Can you work these out from the model? Positions are in its coordinate system, mm. Face numbers are marked on the shaded views. A direction names the side the tool comes from. Round coordinates to 2 decimals unless told otherwise and drop trailing zeros. Loops run counter-clockwise (first coordinate to the right, second up) from the corner with the lowest first, then second, coordinate; pieces in that order, holes last. Notation, with made-up numbers: (-33, 72.5) - (-5, 72.5) arc R12 cw to (-5, 79.5) - close; hole circle Ø5 at (89.5, 15.25). An arc over 180 degrees is marked (long way). Answer as CSV lines item,"result".
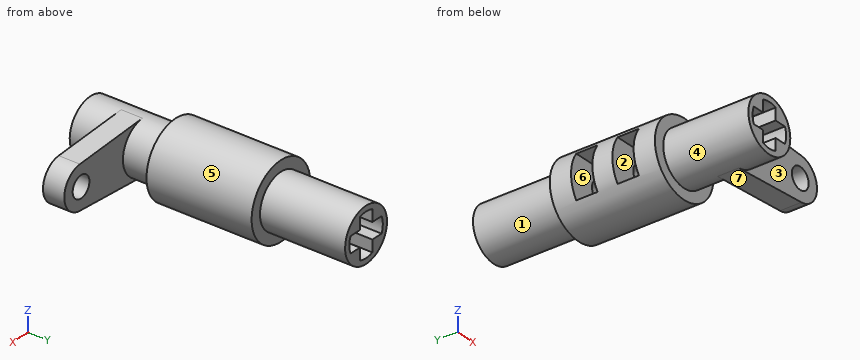
```python
from build123d import *

# Parameters (mm, degrees)
SKETCH_1_R           = 2.5
EXTRUDE_1_DEPTH      = 25.88
EXTRUDE_START        = 3
SKETCH_2_R           = 1
EXTRUDE_2_DEPTH      = 2
CUT_EXTRUDE_1_DEPTH  = 4
CUT_EXTRUDE_START    = 21.88
CUT_EXTRUDE_2_DEPTH  = 4
SKETCH_6_R           = 0.25
CUT_EXTRUDE_3_DEPTH  = 0.25
CUT_EXTRUDE_START_2  = 4.25
SKETCH_7_R           = 0.25
CUT_EXTRUDE_4_DEPTH  = 0.25
EXTRUDE_START_2      = 8
SKETCH_17_R          = 3.5
EXTRUDE_5_DEPTH      = 9.88
SKETCH_18_R          = 1
CUT_EXTRUDE_11_DEPTH = 10
CUT_EXTRUDE_START_3  = 15.88
SKETCH_19_R          = 1
CUT_EXTRUDE_12_DEPTH = 10
SKETCH_22_W          = 4
SKETCH_22_H          = 2
CUT_EXTRUDE_13_DEPTH = 10
CUT_EXTRUDE_14_DEPTH = 2
CUT_EXTRUDE_START_4  = 12
CUT_EXTRUDE_15_DEPTH = 2
SKETCH_25_R          = 1
CUT_EXTRUDE_16_DEPTH = 28.789825476


with BuildPart() as part:
    # 草图1 → 凸台-拉伸1 (new body)
    with BuildSketch(Plane(origin=(0, 0, 0), x_dir=(1, 0, 0), z_dir=(0, 1, 0))):
        with Locations(Location((0, 0, 0), (0, 0, 270))):
            Circle(SKETCH_1_R)
    extrude(amount=EXTRUDE_1_DEPTH)

    # 草图2 → 凸台-拉伸2 (add)
    with BuildSketch(Plane(origin=(0, 0, 0), x_dir=(1, 0, 0), z_dir=(0, 1, 0)).offset(EXTRUDE_START)):
        with BuildLine():
            Line((0.166666667, 2.494438258), (7.633333333, 1.995550606))
            ThreePointArc((7.633333333, 1.995550606), (9.5, 0), (7.633333333, -1.995550606))
            Line((7.633333333, -1.995550606), (0.166666667, -2.494438258))
            ThreePointArc((0.166666667, -2.494438258), (-2.5, 0), (0.166666667, 2.494438258))
        make_face()
        with Locations(Location((7.5, 0, 0), (0, 0, 270))):
            Circle(SKETCH_2_R, mode=Mode.SUBTRACT)
    extrude(amount=EXTRUDE_2_DEPTH)

    # 草图3 → 切除-拉伸1 (cut)
    with BuildSketch(Plane(origin=(0, 0, 0), x_dir=(1, 0, 0), z_dir=(0, 1, 0))):
        with BuildLine():
            Line((-1.854049622, -0.75), (-0.75, -0.75))
            Line((-0.75, -0.75), (-0.75, -1.854049622))
            ThreePointArc((-0.75, -1.854049622), (0, -2), (0.75, -1.854049622))
            Line((0.75, -1.854049622), (0.75, -0.75))
            Line((0.75, -0.75), (1.854049622, -0.75))
            ThreePointArc((1.854049622, -0.75), (2, 0), (1.854049622, 0.75))
            Line((1.854049622, 0.75), (0.75, 0.75))
            Line((0.75, 0.75), (0.75, 1.854049622))
            ThreePointArc((0.75, 1.854049622), (0, 2), (-0.75, 1.854049622))
            Line((-0.75, 1.854049622), (-0.75, 0.75))
            Line((-0.75, 0.75), (-1.854049622, 0.75))
            ThreePointArc((-1.854049622, 0.75), (-2, 0), (-1.854049622, -0.75))
        make_face()
    extrude(amount=CUT_EXTRUDE_1_DEPTH, mode=Mode.SUBTRACT)

    # 草图5 → 切除-拉伸2 (cut)
    with BuildSketch(Plane(origin=(0, 0, 0), x_dir=(1, 0, 0), z_dir=(0, 1, 0)).offset(CUT_EXTRUDE_START)):
        with BuildLine():
            Line((1.854049622, 0.75), (0.75, 0.75))
            Line((0.75, 0.75), (0.75, 1.854049622))
            ThreePointArc((0.75, 1.854049622), (0, 2), (-0.75, 1.854049622))
            Line((-0.75, 1.854049622), (-0.75, 0.75))
            Line((-0.75, 0.75), (-1.854049622, 0.75))
            ThreePointArc((-1.854049622, 0.75), (-2, 0), (-1.854049622, -0.75))
            Line((-1.854049622, -0.75), (-0.75, -0.75))
            Line((-0.75, -0.75), (-0.75, -1.854049622))
            ThreePointArc((-0.75, -1.854049622), (0, -2), (0.75, -1.854049622))
            Line((0.75, -1.854049622), (0.75, -0.75))
            Line((0.75, -0.75), (1.854049622, -0.75))
            ThreePointArc((1.854049622, -0.75), (2, 0), (1.854049622, 0.75))
        make_face()
    extrude(amount=CUT_EXTRUDE_2_DEPTH, mode=Mode.SUBTRACT)

    # 草图6 → 切除-拉伸3 (cut)
    with BuildSketch(Plane(origin=(0, 0, 0), x_dir=(1, 0, 0), z_dir=(0, 1, 0)).offset(CUT_EXTRUDE_START)):
        with Locations(Location((0.75, 0, 0), (0, 0, 270))):
            Circle(SKETCH_6_R)
    extrude(amount=-CUT_EXTRUDE_3_DEPTH, mode=Mode.SUBTRACT)

    # 草图7 → 切除-拉伸4 (cut)
    with BuildSketch(Plane(origin=(0, 0, 0), x_dir=(1, 0, 0), z_dir=(0, 1, 0)).offset(CUT_EXTRUDE_START_2)):
        with Locations(Location((0.75, 0, 0), (0, 0, 270))):
            Circle(SKETCH_7_R)
    extrude(amount=-CUT_EXTRUDE_4_DEPTH, mode=Mode.SUBTRACT)

    # 草图17 → 凸台-拉伸5 (add)
    with BuildSketch(Plane(origin=(0, 0, 0), x_dir=(1, 0, 0), z_dir=(0, 1, 0)).offset(EXTRUDE_START_2)):
        with Locations(Location((0, 0, 0), (0, 0, 270))):
            Circle(SKETCH_17_R)
    extrude(amount=EXTRUDE_5_DEPTH)

    # 草图18 → 切除-拉伸11 (cut)
    with BuildSketch(Plane(origin=(0, 0, 0), x_dir=(1, 0, 0), z_dir=(0, 1, 0))):
        with Locations(Location((0, 0, 0), (0, 0, 270))):
            Circle(SKETCH_18_R)
    extrude(amount=CUT_EXTRUDE_11_DEPTH, mode=Mode.SUBTRACT)

    # 草图19 → 切除-拉伸12 (cut)
    with BuildSketch(Plane(origin=(0, 0, 0), x_dir=(1, 0, 0), z_dir=(0, 1, 0)).offset(CUT_EXTRUDE_START_3)):
        with Locations(Location((0, 0, 0), (0, 0, 270))):
            Circle(SKETCH_19_R)
    extrude(amount=CUT_EXTRUDE_12_DEPTH, mode=Mode.SUBTRACT)

    # 草图22 → 切除-拉伸13 (cut)
    with BuildSketch(Plane(origin=(0, 0, 0), x_dir=(0, 0, -1), z_dir=(1, 0, 0))):
        with Locations((0, 14.88)):
            Rectangle(SKETCH_22_W, SKETCH_22_H)
        with Locations((0, 11)):
            Rectangle(SKETCH_22_W, SKETCH_22_H)
    extrude(amount=-CUT_EXTRUDE_13_DEPTH, mode=Mode.SUBTRACT)

    # 草图23 → 切除-拉伸14 (cut)
    with BuildSketch(Plane(origin=(0, 0, 0), x_dir=(1, 0, 0), z_dir=(0, 1, 0)).offset(CUT_EXTRUDE_START_3)):
        Polygon((-2.309401077, 0), (-1.154700538, -2), (1.154700538, -2), (2.309401077, 0), (1.154700538, 2), (-1.154700538, 2), align=None)
    extrude(amount=-CUT_EXTRUDE_14_DEPTH, mode=Mode.SUBTRACT)

    # 草图24 → 切除-拉伸15 (cut)
    with BuildSketch(Plane(origin=(0, 0, 0), x_dir=(1, 0, 0), z_dir=(0, 1, 0)).offset(CUT_EXTRUDE_START_4)):
        Polygon((-2.309401077, 0), (-1.154700538, -2), (1.154700538, -2), (2.309401077, 0), (1.154700538, 2), (-1.154700538, 2), align=None)
    extrude(amount=-CUT_EXTRUDE_15_DEPTH, mode=Mode.SUBTRACT)

    # 草图25 → 切除-拉伸16 (cut, through all)
    with BuildSketch(Plane(origin=(0, 0, 0), x_dir=(1, 0, 0), z_dir=(0, 1, 0))):
        with Locations(Location((0, 0, 0), (0, 0, 270))):
            Circle(SKETCH_25_R)
    extrude(amount=CUT_EXTRUDE_16_DEPTH, mode=Mode.SUBTRACT)


solid = part.part
```
Q1. I'm going to push flat-ended pins straight in: pin 1 Ø0.9 at (y, z) = (3, 1.5) entering from -X; pin 2 Ø1 at (y, z) = (4, -1) entering from -X; pin 3 Ø3 at (x, z) = (4, 1.5) entering from -Y; pin 4 Ø3.5 at (x, z) = (-0.5, 0) entering from -Y. Where does each tip first touch, or does it pass through?
Checks:
pin 1,"x = -2.27"
pin 2,"x = -2.45"
pin 3,"y = 3"
pin 4,"y = 0"
Q2. Imagine slicing it at A-A (y = 22.75). Write out the boundary of the cut face in (x, z).
Checks:
outline,"circle Ø5 at (0, 0); hole (-1.85, -0.75) - (-0.75, -0.75) - (-0.75, -1.85) arc R2 ccw to (0.75, -1.85) - (0.75, -0.75) - (1.85, -0.75) arc R2 ccw to (1.85, 0.75) - (0.75, 0.75) - (0.75, 1.85) arc R2 ccw to (-0.75, 1.85) - (-0.75, 0.75) - (-1.85, 0.75) arc R2 ccw to start"
Q3. Imagine slicing it at D-D (y = 11.5). Write out the boundary of the cut face in (x, z).
Checks:
outline,"(-2.87, -2) arc R3.5 ccw (long way) to (-2.87, 2) - (1.15, 2) - (2.31, 0) - (1.15, -2) - close"
Q4. Imagine slicing it at B-B (x = 7). Write out the boundary of the cut face in (y, z), then the cut area to 3 significant figures.
Checks:
outline,"(3, -2.04) - (5, -2.04) - (5, -0.87) - (3, -0.87) - close; (3, 0.87) - (5, 0.87) - (5, 2.04) - (3, 2.04) - close"
area,"4.69 mm²"
Q5. On a 3-axis mill with a long thin cutter (end or side, diameter ignored), from which of +Z, -Z, +X, -X, +Y, -Y can I reach the whole of each face in a straight line? I mean the marked faces 4, 5, 6 and 7. Say none if no direction works.
Checks:
face 4,"none"
face 5,"+Y"
face 6,"-X"
face 7,"-Z, +X, -Y"
Q6. If I drill on line 1 along Y through (x, z) = (1, -1.25); line 2 along Y through (x, z) = (-2.5, 0.75); line 3 along X through (y, z) = (8.5, 0), over which ranges is the centre line in solid material (lowest first)? Write a range as [from, to].
Checks:
line 1,"[0, 10], [12, 13.88], [15.88, 25.88]"
line 2,"[8, 10], [12, 13.88], [15.88, 17.88]"
line 3,"[-3.5, -1], [1, 3.5]"
Q7. We'd pull the mould along Y, two halves only. Please class the marked faces 1, 2 and 3: pulls with the +Y half, pulls with the -Y half, needs draft (parallel to the pull), parting line crosses it, or undercut.
Checks:
face 1,"needs draft"
face 2,"undercut"
face 3,"pulls with the -Y half"
